Print and shaded views of the part. All mm, measured from the part's lowest x, y and z. A direction names the side the tool comes from. Round coordinates to 2 decimals unless told otherwise and drop trailing zeros. Loops run counter-clockwise (first coordinate to the right, second up) from the corner with the lowest first, then second, coordinate; pieces in that order, holes last. Notation, with made-up numbers: (79, 52.5) - (87, 52.5) arc R18 ccw to (87, 84.5) - close; hole circle Ø8 at (57.5, -24.75). An arc over 180 degrees is marked (long way). Use one line per item in the form item = value.
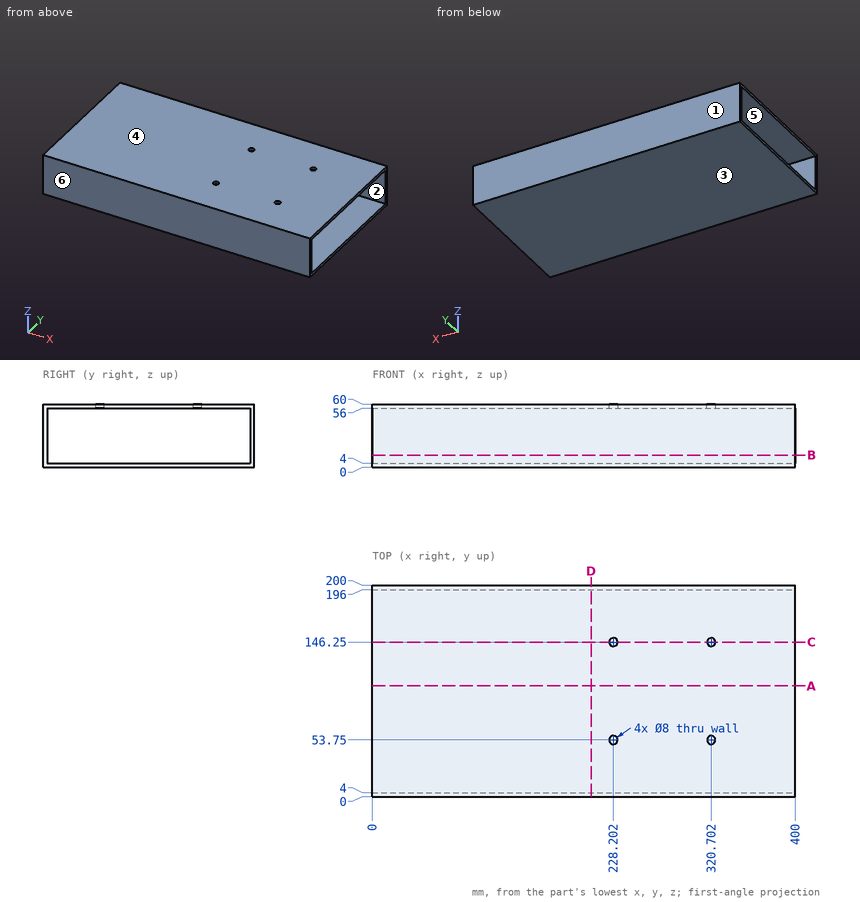
1) Slice it at C-C (y = 146.25). Write the cut outline in (x, z), plus the area to 3 significant figures.
Report:
outline = (0, 0) - (400, 0) - (400, 4) - (0, 4) - close; (0, 56) - (224.2, 56) - (224.2, 60) - (0, 60) - close; (232.2, 56) - (316.7, 56) - (316.7, 60) - (232.2, 60) - close; (324.7, 56) - (400, 56) - (400, 60) - (324.7, 60) - close
area = 3,140 mm^2
2) Tool access for the marked faces 5 and 6: list every direction of +Z, -Z, +X, -X, +Y, -Y with a clear straight run to the whole face (end or side of a thin tool).
Report:
face_5 = +X, -X
face_6 = +Z, -Z, +X, -X, -Y
3) Two-plate mould, pull along Z, no slides. Class the marked faces 1, 2, 3 and 4: +Z half, -Z half, draft (parallel to the pull), parting line (faces both ways), or undercut.
Report:
face_1 = draft
face_2 = undercut
face_3 = -Z half
face_4 = +Z half
4) Slice it at A-A (y = 105). Write the cut outline in (x, z), plus the area to 3 significant figures.
Report:
outline = (0, 0) - (400, 0) - (400, 4) - (0, 4) - close; (0, 56) - (400, 56) - (400, 60) - (0, 60) - close
area = 3,200 mm^2
5) Slice it at B-B (z = 11.5). Write the cut outline in (x, y), plus the area to 3 significant figures.
Report:
outline = (0, 0) - (400, 0) - (400, 4) - (0, 4) - close; (0, 196) - (400, 196) - (400, 200) - (0, 200) - close
area = 3,200 mm^2
6) Drill centre lines: probe 1 along X at (y, z) = (53, 57); probe 2 along X at (y, z) = (146, 59); probe 3 along Y at (x, z) = (179, 20). Where is each one in solid material? Low to high.
Report:
probe_1 = 0 to 224.27, 232.13 to 316.77, 324.63 to 400
probe_2 = 0 to 224.21, 232.19 to 316.71, 324.69 to 400
probe_3 = 0 to 4, 196 to 200
7) Flat gauge pin, fed straight in: pin 1 (5 mm diameter, centred on x = 320.7, y = 146.25, fed in from +Z). Where does the tip first touch, or does it go through?
Report:
pin_1 = 4
8) Slice it at D-D (x = 207). Write the cut outline in (y, z).
Report:
outline = (0, 0) - (200, 0) - (200, 60) - (0, 60) - close; hole (4, 4) - (196, 4) - (196, 56) - (4, 56) - close
